```python
from build123d import *

# Parameters (mm, degrees)
F0_W     = 177.8
F0_H     = 177.8
F1_DEPTH = 47.625
F4_DEPTH = 177.801
F5_DEPTH = 177.801


# Not quite as in the source:
# - ends of sketch curves that miss each other by under 0.0002 mm in the source are joined


with BuildPart() as f1:
    # F0 (on Top) → F1 (new body)
    with BuildSketch(Plane.XY):
        with Locations((-88.9, 88.9)):
            Rectangle(F0_W, F0_H)
    extrude(amount=F1_DEPTH)

    # F3 (on face) → F4 (cut, through all)
    with BuildSketch(Plane(origin=(-177.8, 0, 0), x_dir=(0, -1, 0), z_dir=(-1, 0, 0))):
        Polygon((-177.8, 47.625), (-177.8, 19.0884657204), (-89.0196708441, 47.625), align=None)
        Polygon((-88.7803285837, 47.625), (2.861e-07, 19.0884657204), (0, 47.625), align=None)
    extrude(amount=-F4_DEPTH, mode=Mode.SUBTRACT)

    # F2 (on face) → F5 (cut, through all)
    with BuildSketch(Plane.XZ):
        Polygon((-177.8, 19.05), (-88.9, 47.625), (-177.8, 47.625), align=None)
        Polygon((-88.9, 47.625), (0, 19.05), (0, 47.625), align=None)
    extrude(amount=-F5_DEPTH, mode=Mode.SUBTRACT)


solid = f1.part
```
Could you check a few things on this model? Use its own coordinates, in mm. Coordinates: 2 decimals unless noted, no trailing zeros. Loops run counter-clockwise (first coordinate to the right, second up) from the corner with the lowest first, then second, coordinate; pieces in that order, holes last. Notation, with made-up numbers: M -4.75,-38 L 31.25,-38 A12 cw 31.25,-29 Z; hole C 15.25,3 d9. An arc over 180 degrees is marked long. Put each result on its own line as item: value. Start each with the question number.
(1) Suppose I cut it at D-D on z = 27.5. Please give me the cut outline in (x, y).
(2) Suppose I cut it at B-B on x = -100. Please give me the cut outline in (y, z).
(3) Will these pins go through, and if not, where does the flat tip stop? P1, Ø2, axis at x = -72.5, y = 126, coming from the +Z side; P2, Ø4, axis at x = -72.5, y = 60.5, coming from the +Z side.
(4) I need wall thicknesses on line 1 (Z direction, x = -158.5, y = 143); line 2 (Z direction, x = -100, y = 29.5). Which ranges of each line are inside material? Lowest first, please. Write a range as from..to.
(5) Suppose I cut it at A-A on y = 39.5. Please give me the cut outline in (x, z).
(6) Suppose I cut it at C-C on z = 39. Please give me the cut outline in (x, y).
Solutions:
1. outline: M -151.51,26.17 L -26.29,26.17 L -26.29,151.63 L -151.51,151.63 Z
2. outline: M 0,0 L 177.8,0 L 177.8,19.09 L 100.12,44.06 L 77.68,44.06 L 0,19.09 Z
3. P1: stops at z = 36.06
3. P2: stops at z = 39.18
4. line 1: z = 0..25.25
4. line 2: z = 0..28.57
5. outline: M -177.8,0 L 0,0 L 0,19.05 L -39.62,31.78 L -138.18,31.78 L -177.8,19.05 Z
6. outline: M -115.73,61.95 L -62.07,61.95 L -62.07,115.85 L -115.73,115.85 Z
